Here's how the part is built. I have some questions about the finished solid (model axes, mm). A direction names the side the tool comes from. Round coordinates to 2 decimals unless told otherwise and drop trailing zeros. Write each loop counter-clockwise with the first axis right and the second up, starting at its lowest first coordinate (ties: lowest second). Pieces come first, ordered by that corner, then holes. Notation, with made-up numbers: (7.25, -29) -> (29.25, -29) arc R11 ccw to (29.25, -13) -> close; hole circle Ø2 at (2.25, 46). An arc over 180 degrees is marked (long way). Answer in a Markdown table with one row per item.
from build123d import *

# Parameters (mm, degrees)
SKETCH_1_W             = 80
SKETCH_1_H             = 80
EXTRUDE_1_DEPTH        = 12
HOLE_WIZARD_M121_D     = 10.2
HOLE_WIZARD_M121_DEPTH = 12
SKETCH_12_R            = 4.5
CUT_EXTRUDE_1_DEPTH    = 13
SKETCH_13_R            = 7.5
CUT_EXTRUDE_2_DEPTH    = 9


with BuildPart() as part:
    # Эскиз1 → Бобышка-Вытянуть1 (new body)
    with BuildSketch(Plane(origin=(0, 0, 0), x_dir=(1, 0, 0), z_dir=(0, 1, 0))):
        Rectangle(SKETCH_1_W, SKETCH_1_H)
    extrude(amount=EXTRUDE_1_DEPTH)

    # Отверстие обработанное метчиком M121
    with Locations(Plane(origin=(0, 12, 0), x_dir=(1, 0, 0), z_dir=(0, 1, 0))):
        with Locations((0, 0)):
            Hole(HOLE_WIZARD_M121_D / 2, depth=HOLE_WIZARD_M121_DEPTH)

    # Эскиз12 → Вырез-Вытянуть1 (cut, through all)
    with BuildSketch(Plane(origin=(0, 12, 0), x_dir=(1, 0, 0), z_dir=(0, 1, 0))):
        with Locations(Location((-20, 20, 0), (0, 0, 270))):  # turned: the seam where the file's is
            Circle(SKETCH_12_R)
        with Locations(Location((20, 20, 0), (0, 0, 270))):  # turned: the seam where the file's is
            Circle(SKETCH_12_R)
        with Locations(Location((20, -20, 0), (0, 0, 270))):  # turned: the seam where the file's is
            Circle(SKETCH_12_R)
        with Locations(Location((-20, -20, 0), (0, 0, 270))):  # turned: the seam where the file's is
            Circle(SKETCH_12_R)
    extrude(amount=-CUT_EXTRUDE_1_DEPTH, mode=Mode.SUBTRACT)

    # Эскиз13 → Вырез-Вытянуть2 (cut)
    with BuildSketch(Plane(origin=(0, 12, 0), x_dir=(1, 0, 0), z_dir=(0, 1, 0))):
        with Locations(Location((-20, 20, 0), (0, 0, 270))):  # turned: the seam where the file's is
            Circle(SKETCH_13_R)
        with Locations(Location((20, 20, 0), (0, 0, 270))):  # turned: the seam where the file's is
            Circle(SKETCH_13_R)
        with Locations(Location((20, -20, 0), (0, 0, 270))):  # turned: the seam where the file's is
            Circle(SKETCH_13_R)
        with Locations(Location((-20, -20, 0), (0, 0, 270))):  # turned: the seam where the file's is
            Circle(SKETCH_13_R)
    extrude(amount=-CUT_EXTRUDE_2_DEPTH, mode=Mode.SUBTRACT)


solid = part.part
1) I need wall thicknesses on line 1 (X direction, y = 0.6, z = -20); line 2 (X direction, y = 6, z = 20); line 3 (Z direction, x = 19, y = 9.75). Which ranges of each line are inside material? Lowest first, please. Write a range as [from, to].
Response:
| item | result |
|---|---|
| line 1 | x = [-40, -24.5], [-15.5, 15.5], [24.5, 40] |
| line 2 | x = [-40, -27.5], [-12.5, 12.5], [27.5, 40] |
| line 3 | z = [-40, -27.43], [-12.57, 12.57], [27.43, 40] |
2) I want a section at C-C, the plane x = -20. List the corners of the cut face in (y, z) for me, and give its area (3 significant figures).
Response:
| item | result |
|---|---|
| outline | (0, -40) -> (12, -40) -> (12, -27.5) -> (3, -27.5) -> (3, -24.5) -> (0, -24.5) -> close; (0, -15.5) -> (3, -15.5) -> (3, -12.5) -> (12, -12.5) -> (12, 12.5) -> (3, 12.5) -> (3, 15.5) -> (0, 15.5) -> close; (0, 24.5) -> (3, 24.5) -> (3, 27.5) -> (12, 27.5) -> (12, 40) -> (0, 40) -> close |
| area | 636 mm^2 |
3) I want a section at D-D, the plane y = 5. List the corners of the cut face in (x, z) for me, and give its area (3 significant figures).
Response:
| item | result |
|---|---|
| outline | (-40, -40) -> (40, -40) -> (40, 40) -> (-40, 40) -> close; hole circle Ø15 at (-20, -20); hole circle Ø15 at (-20, 20); hole circle Ø10.2 at (0, 0); hole circle Ø15 at (20, -20); hole circle Ø15 at (20, 20) |
| area | 5,610 mm^2 |
4) Which directions (+Z, -Z, +X, -X, +Y, -Y) give clear straight access to the entire face, cutting with the end or side of a thin tool? Please do faces 4 (the face through (20, 3, 25)), 5 (the face through (-40, 6, 1)).
Response:
| item | result |
|---|---|
| face 4 | +Y |
| face 5 | +Z, -Z, -X, +Y, -Y |
5) I want a section at A-A, the plane z = 20. List the corners of the cut face in (x, y) for me, and give its area (3 significant figures).
Response:
| item | result |
|---|---|
| outline | (-40, 0) -> (-24.5, 0) -> (-24.5, 3) -> (-27.5, 3) -> (-27.5, 12) -> (-40, 12) -> close; (-15.5, 0) -> (15.5, 0) -> (15.5, 3) -> (12.5, 3) -> (12.5, 12) -> (-12.5, 12) -> (-12.5, 3) -> (-15.5, 3) -> close; (24.5, 0) -> (40, 0) -> (40, 12) -> (27.5, 12) -> (27.5, 3) -> (24.5, 3) -> close |
| area | 636 mm^2 |
6) I want a section at B-B, the plane x = 0. List the corners of the cut face in (y, z) for me.
Response:
| item | result |
|---|---|
| outline | (0, -40) -> (12, -40) -> (12, -5.1) -> (0, -5.1) -> close; (0, 5.1) -> (12, 5.1) -> (12, 40) -> (0, 40) -> close |
7) For pin 1 (7.5 mm diameter, centred on x = -22.5, z = -19.5, fed in from +Y); pin 2 (13.5 mm diameter, centred on x = 20, z = 20, fed in from -Y); pin 3 (8 mm diameter, centred on x = -20, z = -20, fed in from -Y), each with a flat end and sliding along its axis, tell me the tip position at first contact or that it passes through.
Response:
| item | result |
|---|---|
| pin 1 | stops at y = 3 |
| pin 2 | stops at y = 0 |
| pin 3 | passes through |
8) We'd pull the mould along X, two halves only. Please class faces 1 (the face through (-19.67, 7.563, 12.507)), 2 (the face through (40, 6, 1)), 3 (the face through (-1, 6, 40)): +X half, -X half, draft (parallel to the pull), parting line (faces both ways), or undercut.
Response:
| item | result |
|---|---|
| face 1 | undercut |
| face 2 | +X half |
| face 3 | draft |
